Can you work these out from the drawing? Everything is in mm from the part's minimum corner. A direction names the side the tool comes from. Coordinates: 2 decimals unless noted, no trailing zeros. Write each loop counter-clockwise with the first axis right and the second up, starting at its lowest first coordinate (ties: lowest second). Pieces come first, ordered by that corner, then holes. Notation, with made-up numbers: (10.5, 50.25) - (54.5, 50.25) arc R23 ccw to (54.5, 74.25) - close; hole circle Ø9 at (38.25, -12.75). An arc over 180 degrees is marked (long way). One line per question, with ' | ' between items. Start each with the question number.
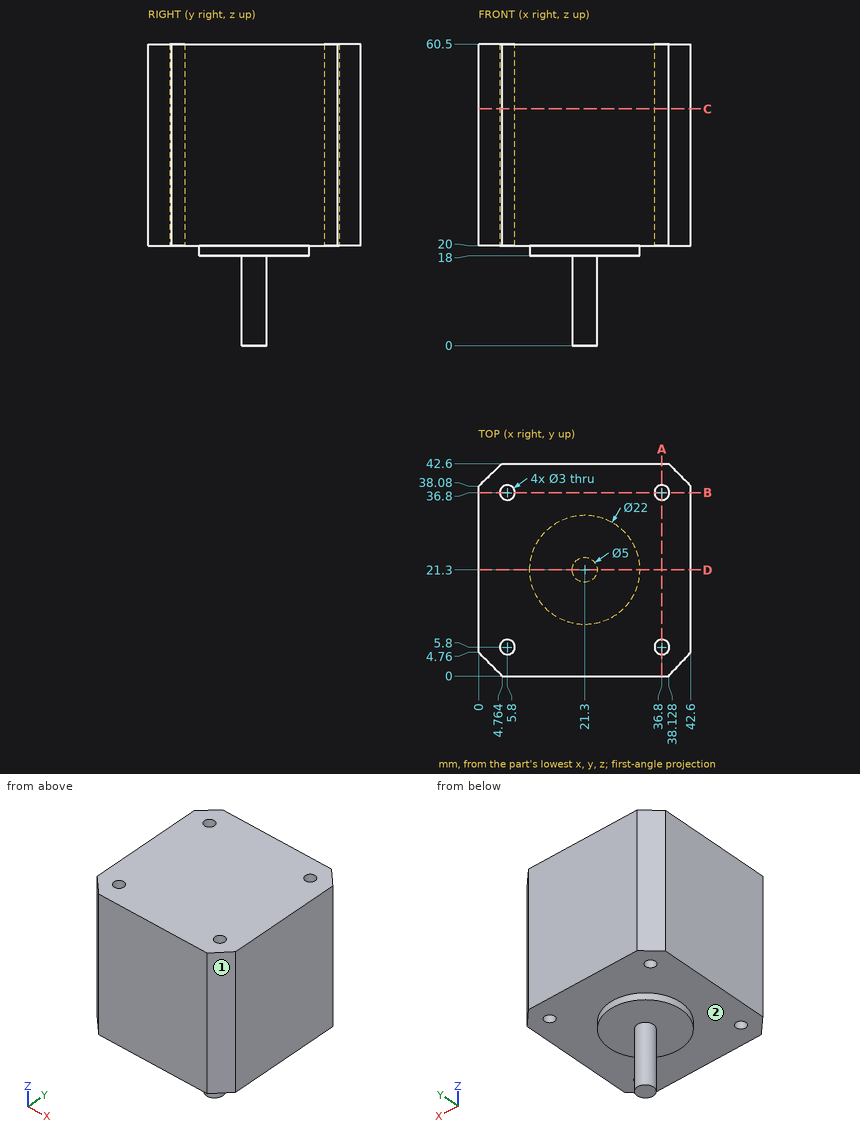
(1) Which directions (+Z, -Z, +X, -X, +Y, -Y) give clear straight access to the entire face, cutting with the end or side of a thin tool? Please do the marked faces 1 and 2.
(2) I'm going to push flat-ended pins straight in: pin 1 (3 mm diameter, centred on x = 28, y = 25, fed in from -Z); pin 2 (2 mm diameter, centred on x = 7, y = 21.5, fed in from -Z); pin 3 (2.5 mm diameter, centred on x = 5.8, y = 36.8, fed in from -Z). Where does each tip first touch, or does it pass through?
(3) If we section it at C-C on z = 47.5: List the corners of the cut face in (x, y) for me (1 decimal).
(4) If I drill on probe 1 along Y at (x, z) = (36.8, 41.5); probe 2 along Y at (x, z) = (5, 36); probe 3 along X at (y, z) = (6.5, 45.5) (1 decimal), over which ranges is the centre line in solid material (lowest first)?
(5) If we section it at D-D on y = 21.3: List the corners of the cut face in (x, z) for me.
(6) If we section it at A-A on x = 36.8: List the corners of the cut face in (y, z) for me, plus the area to 3 significant figures.
Values:
1) face 1: +Z, -Z, +X, -Y | face 2: -Z
2) pin 1: z = 18 | pin 2: z = 20 | pin 3: through
3) outline: (0, 4.8) - (4.8, 0) - (38.1, 0) - (42.6, 4.8) - (42.6, 38.1) - (38.1, 42.6) - (4.8, 42.6) - (0, 38.1) - close; hole circle Ø3 at (5.8, 5.8); hole circle Ø3 at (5.8, 36.8); hole circle Ø3 at (36.8, 5.8); hole circle Ø3 at (36.8, 36.8)
4) probe 1: 0 to 4.3, 7.3 to 35.3, 38.3 to 42.6 | probe 2: 0 to 4.53, 7.07 to 35.53, 38.07 to 42.6 | probe 3: 0 to 4.5, 7.1 to 35.5, 38.1 to 42.6
5) outline: (0, 20) - (10.3, 20) - (10.3, 18) - (18.8, 18) - (18.8, 0) - (23.8, 0) - (23.8, 18) - (32.3, 18) - (32.3, 20) - (42.6, 20) - (42.6, 60.5) - (0, 60.5) - close
6) outline: (0, 20) - (4.3, 20) - (4.3, 60.5) - (0, 60.5) - close; (7.3, 20) - (35.3, 20) - (35.3, 60.5) - (7.3, 60.5) - close; (38.3, 20) - (42.6, 20) - (42.6, 60.5) - (38.3, 60.5) - close | area: 1,480 mm2
